Verification items for the finished model (mm, model axes). Face numbers are marked on the shaded views. Coordinates: 2 decimals unless noted, no trailing zeros. Order: outer loops, then holes, each group sorted by start corner. A loop starts at its lowest first (then second) coordinate and runs counter-clockwise, first axis right, second up. Notation, with made-up numbers: M -24,46.25 L -6,46.25 A20 cw -6,66.25 Z; hole C 10,-18.5 d6. An arc over 180 degrees is marked long. Write item = value, one per line.
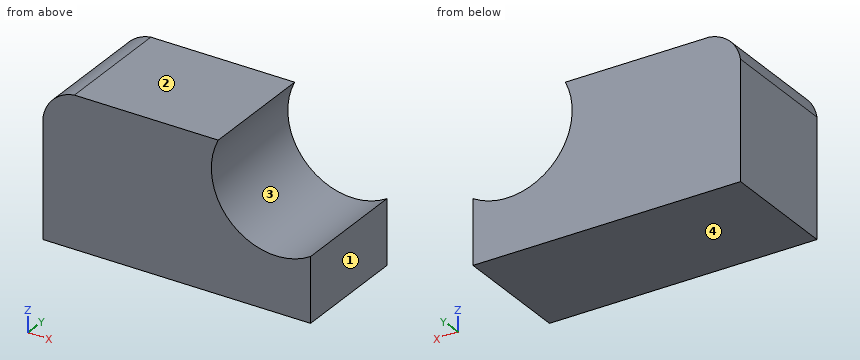
```python
from build123d import *

# Parameters (mm, degrees)
F0_W     = 57.15
F0_H     = 31.75
F1_DEPTH = 25.4
F3_DEPTH = 25.4
F5_R     = 13.8731046092
F6_DEPTH = 25.4


# Not quite as in the source:
# - a feature names something its author has since deleted; it is built from what else it names


with BuildPart() as f1:
    # F0 (on Front) → F1 (new body)
    with BuildSketch(Plane.XZ):
        with Locations((28.575, 15.875)):
            Rectangle(F0_W, F0_H)
    extrude(amount=F1_DEPTH)

    # F2 (on face) → F3 (cut)
    with BuildSketch(Plane.XZ.offset(25.4)):
        with BuildLine():
            ThreePointArc((0, 25.186264758), (2.2625309899, 29.5850653675), (6.7101765828, 31.75))
            Line((6.7101765828, 31.75), (0, 31.75))
            Line((0, 31.75), (0, 25.186264758))
        make_face()
    extrude(amount=-F3_DEPTH, mode=Mode.SUBTRACT)

    # F5 (on face) → F6 (cut)
    with BuildSketch(Plane.XZ.offset(25.4)):
        with Locations((49.8321466148, 25.5351066589)):
            Circle(F5_R)
    extrude(amount=-F6_DEPTH, mode=Mode.SUBTRACT)


solid = f1.part
```
Item 1: Sectioned sample at C-C, the plane x = 51.5. Enter the section's corners in (y, z).
Report:
outline = M -25.4,0 L 0,0 L 0,11.76 L -25.4,11.76 Z
Item 2: Gauge pin test, flat ends, axial feed: pin 1 (8 mm diameter, centred on y = -20.5, z = 14, fed in from +X); pin 2 (1.5 mm diameter, centred on x = 40.5, y = -14.5, fed in from +Z). Record the tip position at first contact, or that the pin passes through.
Report:
pin_1 = 57.15
pin_2 = 16.01
Item 3: Sectioned sample at B-B, the plane z = 13. Enter the section's corners in (x, y).
Report:
outline = M 0,-25.4 L 43.89,-25.4 L 43.89,0 L 0,0 Z; M 55.78,-25.4 L 57.15,-25.4 L 57.15,0 L 55.78,0 Z
Item 4: Sectioned sample at D-D, the plane z = 23. Enter the section's corners in (x, y).
Report:
outline = M 0,-25.4 L 36.19,-25.4 L 36.19,0 L 0,0 Z
Item 5: Sectioned sample at A-A, the plane y = -4.5. Enter the section's corners in (x, z), then the cut area to 3 significant figures.
Report:
outline = M 0,0 L 57.15,0 L 57.15,13.75 A13.87 cw 37.43,31.75 L 6.71,31.75 A7.83 ccw 0,25.19 Z
area = 1,430 mm^2
Item 6: Scan lines: L1, parallel to Z at x = 50, y = -10; L2, parallel to Z at x = 38, y = -17; L3, parallel to X at y = -12, z = 13. Record each from-to range of solid material in increasing order. Write a range as from..to.
Report:
L1 = 0..11.66
L2 = 0..18.29
L3 = 0..43.89, 55.78..57.15
Item 7: Release check for a two-part mould opening along Z. For the marked faces 1, 2, 3 and 4 record: pulls with the +Z half, pulls with the -Z half, needs draft (parallel to the pull), parting line crosses it, or undercut.
Report:
face_1 = needs draft
face_2 = pulls with the +Z half
face_3 = undercut
face_4 = pulls with the -Z half
